Study the drawing (mm; zero at the part's minimum x, y, z) and answer. A direction names the side the tool comes from. Give positions to 0.01 mm unless a question says otherwise; leave off trailing zeros. Loops run counter-clockwise (first coordinate to the right, second up) from the corner with the lowest first, then second, coordinate; pieces in that order, holes last. Notation, with made-up numbers: M 24,-1 L 60,-1 A15 ccw 60,15 Z; hole C 24,18.5 d3. An arc over 180 degrees is marked long. Return JSON: item names as keys, results as strings.
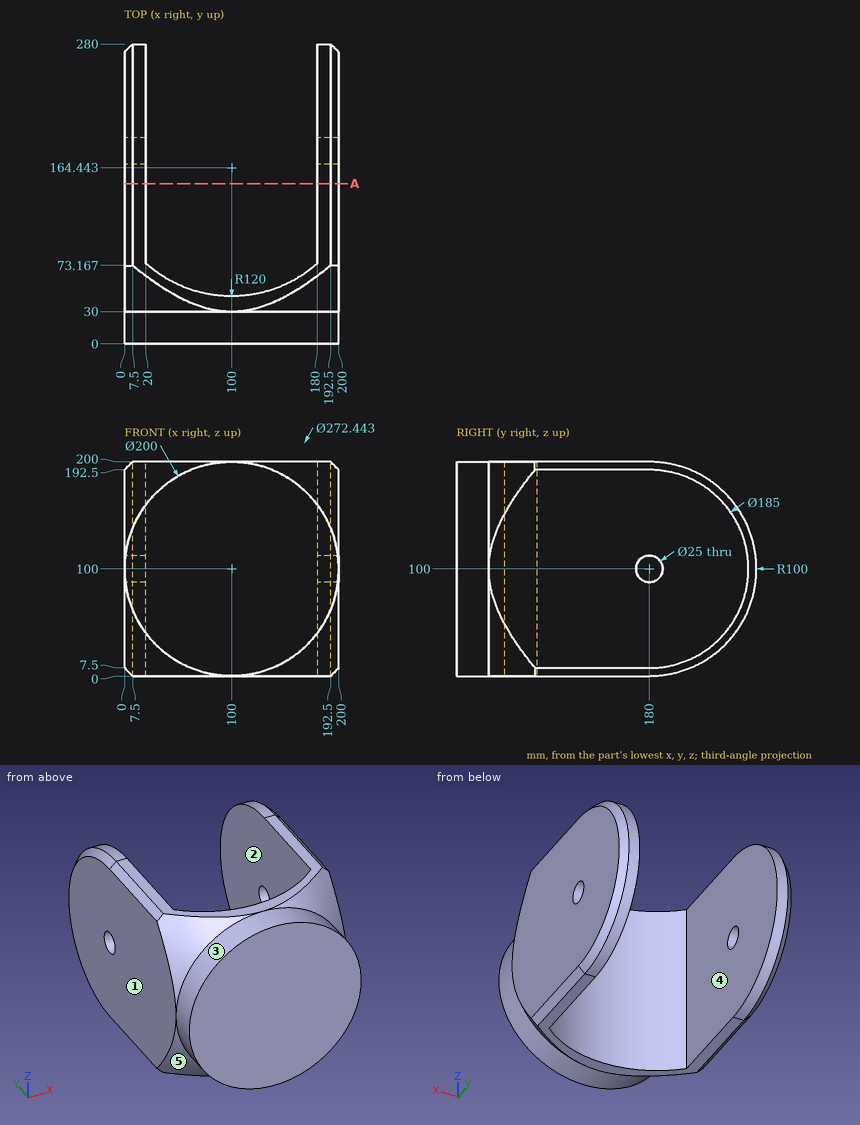
(1) Determine the mould class of the marked faces 3, 4 and 5 for opening direction X: released by +X, released by -X, zero draft, split by the parting line, or undercut.
Values follow:
{"face 3": "split by the parting line", "face 4": "undercut", "face 5": "released by -X"}
(2) Straight lines are drawn through the part: line 1 along X through (y, z) = (196.5, 36); line 2 along Z through (x, y) = (14, 180); line 3 along Y through (x, z) = (185.75, 100). For each, find the intervals that lie inside material, in ascending order.
Values follow:
{"line 1": "0 to 20, 180 to 200", "line 2": "0 to 87.5, 112.5 to 200", "line 3": "0 to 167.5, 192.5 to 280"}
(3) The part is cut by section A-A (y = 149.5). Determine the outline of the cut face in (x, z), and give its area (3 significant figures).
Values follow:
{"outline": "M 0,7.5 L 7.5,0 L 20,0 L 20,200 L 7.5,200 L 0,192.5 Z; M 180,0 L 192.5,0 L 200,7.5 L 200,192.5 L 192.5,200 L 180,200 Z", "area": "7,890 mm²"}
(4) A tool of negligible diameter and unlimited length cuts with its end or side. For the marked faces 1 and 2, from which of +Z, -Z, +X, -X, +Y, -Y can it reach the whole face along a straight path? Write none if from no direction.
Values follow:
{"face 1": "+Z, -Z, -X, +Y, -Y", "face 2": "+Z, -Z, +Y"}
(5) Given pin 1 (20 mm diameter, centred on y = 180, z = 100, fed in from +X); pin 2 (5 mm diameter, centred on x = 120, z = 110, fed in from +Y), each flat-ended and moving along its own axis, determine where each tip first touches the part or whether it passes through.
Values follow:
{"pin 1": "through", "pin 2": "y = 46.57"}
